Autodesk Inventor part; units mm, degrees
ref_plane "YZ Plane" through (0, 0, 0) normal (1, 0, 0) x (0, 1, 0)
ref_plane "XZ Plane" through (0, 0, 0) normal (0, 1, 0) x (-1, 0, 0)
ref_plane "XY Plane" through (0, 0, 0) normal (0, 0, 1) x (1, 0, 0)
sketch "Sketch1" plane through (0, 0, 0) normal (0, 0, 1) x (1, 0, 0)
  circle A0 centre (0, 0) radius 34.798
  circle A1 centre (0, 0) radius 41.275
  line L0 (38.2986, -15.3898) -> (35.2745, -14.5795)
  line L1 (35.2745, -14.5795) -> (37.8384, -5.011)
  line L2 (37.8384, -5.011) -> (40.8624, -5.8213)
  line L3 (0, 0) -> (36.5564, -9.7953) construction
  line L4 (0, 0) -> (34.798, 0) construction
  line L5 (36.5564, -9.7953) -> (39.8686, -10.6828) construction
  dimension "d0" = 69.596
  dimension "d1" = 82.55
  dimension "d2" = 15
  dimension "d3" = 9.906
  dimension "d4" = 3.429
extrude "Extrusion1" add sketch "Sketch1" along normal blind 2.54
extrude "Extrusion2" cut sketch "Sketch1" along normal blind 2.54 contours L0 L1 L2 A1 picked at (37.7926, -9.5555)
pattern_circular "Circular Pattern1" count 3 over 60 about axis through (0, 0, 0) along (0, 0, 1) of "Extrusion2"
mirror "Mirror1" about plane through (0, 0, 0) normal (1, 0, 0) of "Extrusion2", "Circular Pattern1"
sketch "Sketch2" plane through (0, 0, 0) normal (0, 0, -1) x (-1, 0, 0)
  circle A0 centre (0, 0) radius 34.798
  circle A1 centre (0, 0) radius 33.02
  dimension "d12" = 66.04
extrude "Extrusion3" add sketch "Sketch2" against normal blind 5.08
sketch "Sketch3" plane through (0, 0, 0) normal (0, 0, -1) x (-1, 0, 0)
  arc A0 (25.4726, 32.4772) -> (-25.4726, 32.4772) centre (0, 0) ccw
  line L0 (-17.2903, 37.4789) -> (-16.1691, 34.3986)
  line L1 (-16.1691, 34.3986) -> (-9.7247, 36.7442)
  line L2 (-9.7247, 36.7442) -> (-10.8459, 39.8245)
  line L3 (0, 0) -> (-12.9469, 35.5714) construction
  line L4 (-12.9469, 35.5714) -> (-13.8833, 38.8701) construction
  line L5 (0, 0) -> (13.6723, 0) construction
  dimension "d15" = 3.429
  dimension "d16" = 6.858
  dimension "d17" = 110
extrude "Extrusion4" cut sketch "Sketch3" against normal blind 5.08
properties part number "BallastTankMillOutline"
Verification items for the finished model (mm, model axes). A direction names the side the tool comes from. Round coordinates to 2 decimals unless told otherwise and drop trailing zeros. Write each loop counter-clockwise with the first axis right and the second up, starting at its lowest first coordinate (ties: lowest second). Pieces come first, ordered by that corner, then holes.
1. Gauge pin test, flat ends, axial feed: P1, Ø12, axis at x = 16.5, y = 32, coming from the +Z side; P2, Ø2, axis at x = -14, z = 3, coming from the -Y side; P3, Ø2, axis at x = 5.5, z = 4.5, coming from the +Y side. Record the tip position at first contact, or that the pin passes through.
2. Access from +Z, -Z, +X, -X, +Y, -Y to the whole of each face (thin tool, end or side, straight path). Record for faces 1 (the cylindrical face through (35.704, 20.708, 1.252)), 2 (the cylindrical face through (7.54, -33.97, 3.79)), 3 (the flat face through (31.386, 24.381, 1.252)), 4 (the flat face through (-24.381, 31.386, 1.252)), 5 (the flat face through (26.81, 26.71, 1.25)).
3. Draft check along Y on faces 6 (the flat face through (-13, -31, 5.08)), 7 (the cylindrical face through (41.275, 0.082, 1.252)), 8 (the flat face through (-36.574, -9.728, 1.252)), 9 (the cylindrical face through (-31.5, 9.9, 2.5)). Enter one of: +Y half, -Y half, draft (parallel to the pull), parting line (faces both ways), or undercut.
4. Scan lines: L1, parallel to X at y = 23.5, z = 0.3; L2, parallel to Y at x = 0, z = 1.7 (3 decimals); L3, parallel to Y at x = 0, z = 2.75. Record each from-to range of solid material in increasing order.
5. Section check A-A on y = 0. Enter the section's corners in (x, z) (3 decimals).
Answer:
1. P1: stops at z = 5.08
1. P2: stops at y = -39.14
1. P3: stops at y = 34.51
2. face 1: +Z, -Z, +X, +Y
2. face 2: +Z
2. face 3: +Z, -Z, +Y
2. face 4: +Z, -Z, -X
2. face 5: +Z, -Z
3. face 6: draft
3. face 7: parting line
3. face 8: undercut
3. face 9: undercut
4. L1: x = -33.93 to -30.5, -30.02 to -23.2, 23.2 to 30.02, 30.5 to 33.93
4. L2: y = -41.275 to -33.02, 33.02 to 41.275
4. L3: y = -34.8 to -33.02, 33.02 to 34.8
5. outline: (-41.275, 0) - (-33.02, 0) - (-33.02, 5.08) - (-34.798, 5.08) - (-34.798, 2.54) - (-41.275, 2.54) - close; (33.02, 0) - (41.275, 0) - (41.275, 2.54) - (34.798, 2.54) - (34.798, 5.08) - (33.02, 5.08) - close
